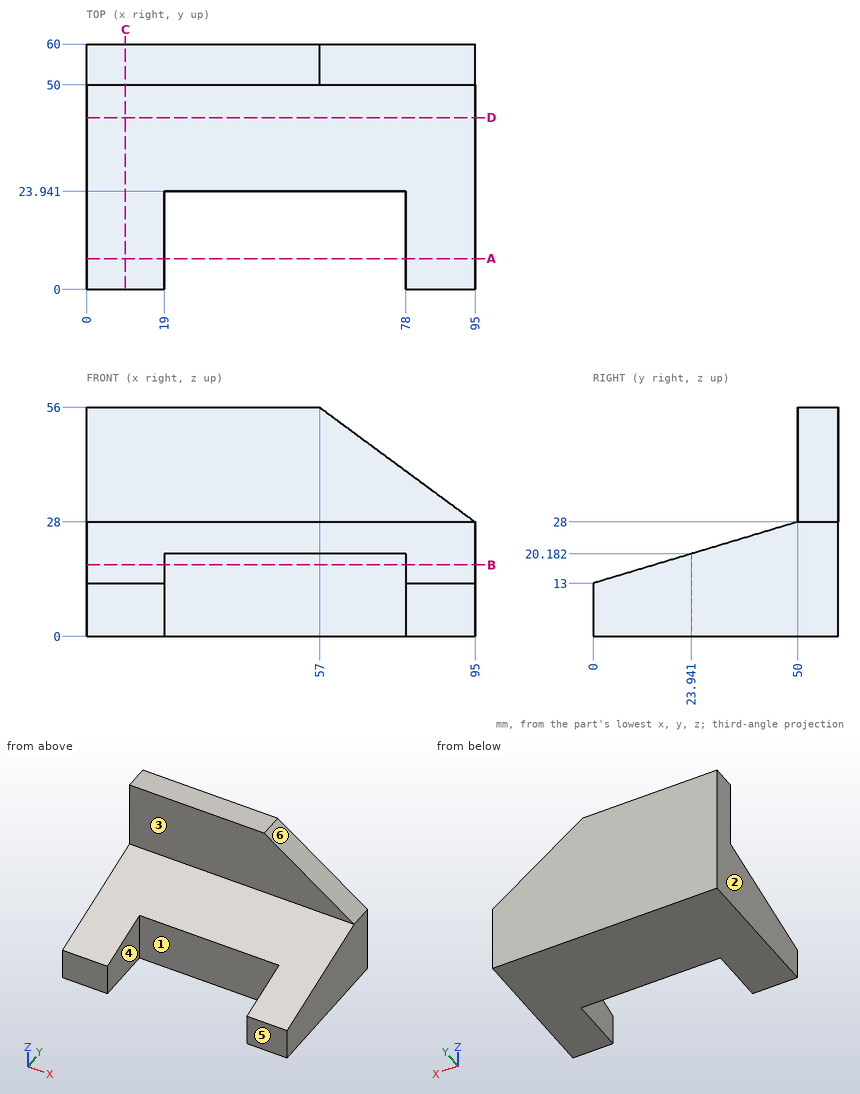
Design review of the part shown in the three views and the two pictorial views. Dimensions are in mm from the part's minimum x, y and z. A direction names the side the tool comes from. Round coordinates to 2 decimals unless told otherwise and drop trailing zeros. Loops run counter-clockwise (first coordinate to the right, second up) from the corner with the lowest first, then second, coordinate; pieces in that order, holes last.
Q1. Add section A-A on y = 7.5. Write out the cut boundary in (x, z), plus the area to 3 significant figures.
Result sheet:
outline: (0, 0) - (19, 0) - (19, 15.25) - (0, 15.25) - close; (78, 0) - (95, 0) - (95, 15.25) - (78, 15.25) - close
area: 549 mm2
Q2. Add section C-C on x = 9.5. Write out the cut boundary in (y, z), plus the area to 4 significant figures.
Result sheet:
outline: (0, 0) - (60, 0) - (60, 56) - (50, 56) - (50, 28) - (0, 13) - close
area: 1,585 mm2
Q3. Add section B-B on z = 17.5. Write out the cut boundary in (x, y).
Result sheet:
outline: (0, 15) - (19, 15) - (19, 23.94) - (78, 23.94) - (78, 15) - (95, 15) - (95, 60) - (0, 60) - close
Q4. Mouldability with a two-part tool opening along X and no side actions: class the marked faces 4, 5 and 6 as +X half, -X half, draft (parallel to the pull), parting line (faces both ways), or undercut.
Result sheet:
face 4: undercut
face 5: draft
face 6: +X half
Q5. Insertion check: pin 1 Ø1.5 at (x, y) = (54, 23.5) entering from -Z; pin 2 Ø5 at (x, z) = (33, 42) entering from -Y; pin 3 Ø3 at (y, z) = (7.5, 18) entering from -X; pin 4 Ø1.5 at (y, z) = (53.5, 41.5) entering from +X. Each pin has a flat end and moves straight along its axis. Give the tip position at first contact, or say it passes through.
Result sheet:
pin 1: stops at z = 0
pin 2: stops at y = 50
pin 3: passes through
pin 4: stops at x = 77.7
Q6. To check wall thickness, follow line 1 along Y through (x, z) = (43.5, 49); line 2 along Y through (x, z) = (31.5, 5); line 3 along Z through (x, y) = (36, 36.5). State the ranges of each line that lie inside material, in increasing order.
Result sheet:
line 1: y = 50 to 60
line 2: y = 23.94 to 60
line 3: z = 0 to 23.95
Q7. Add section D-D on y = 42. Write out the cut boundary in (x, z).
Result sheet:
outline: (0, 0) - (95, 0) - (95, 25.6) - (0, 25.6) - close
Q8. Machinability: for the marked faces 1, 2 and 3, which of the approach directions +Z, -Z, +X, -X, +Y, -Y give a long, thin tool a straight path to every point of the face, cutting with its end or side? Answer none if there is none.
Result sheet:
face 1: +Z, -Z, -Y
face 2: +Z, -Z, -X, +Y, -Y
face 3: +Z, +X, -X, -Y
